```python
from build123d import *

# Parameters (mm, degrees)
CROQUIS1_R              = 3
SALIENTE_EXTRUIR1_DEPTH = 5
CHAFL_N1_SIZE           = 2


with BuildPart() as part:
    # Croquis1 → Saliente-Extruir1 (new body)
    with BuildSketch(Plane(origin=(0, 0, 0), x_dir=(1, 0, 0), z_dir=(0, 1, 0))):
        Polygon((-149.607843137, -39.607843137), (-129.607843137, -19.607843137), (170.392156863, -19.607843137), (190.392156863, -39.607843137), (220.392156863, -39.607843137), (220.392156863, 40.392156863), (-179.607843137, 40.392156863), (-179.607843137, -39.607843137), align=None)
        with Locations(Location((-164.607843137, 20.392156863, 0), (0, 0, 270))):
            Circle(CROQUIS1_R, mode=Mode.SUBTRACT)
        with Locations(Location((-99.607843137, 30.392156863, 0), (0, 0, 270))):
            Circle(CROQUIS1_R, mode=Mode.SUBTRACT)
        with Locations(Location((140.392156863, 30.392156863, 0), (0, 0, 270))):
            Circle(CROQUIS1_R, mode=Mode.SUBTRACT)
        with Locations(Location((20.392156863, 30.392156863, 0), (0, 0, 270))):
            Circle(CROQUIS1_R, mode=Mode.SUBTRACT)
        with Locations(Location((-164.607843137, -19.607843137, 0), (0, 0, 270))):
            Circle(CROQUIS1_R, mode=Mode.SUBTRACT)
        with Locations(Location((205.392156863, 20.392156863, 0), (0, 0, 270))):
            Circle(CROQUIS1_R, mode=Mode.SUBTRACT)
        with Locations(Location((205.392156863, -19.607843137, 0), (0, 0, 270))):
            Circle(CROQUIS1_R, mode=Mode.SUBTRACT)
    extrude(amount=SALIENTE_EXTRUIR1_DEPTH)

    # Chaflán1
    chafl_n1_edges = [part.edges().sort_by_distance(p)[0] for p in [
        (-139.607843137, 5, 29.607843137),
        (20.392156863, 5, 19.607843137),
        (180.392156863, 5, 29.607843137),
        (205.392156863, 5, 39.607843137),
        (220.392156863, 5, -0.392156863),
        (20.392156863, 5, -40.392156863),
        (-179.607843137, 5, -0.392156863),
        (-164.607843137, 5, 39.607843137),
    ]]
    chamfer(chafl_n1_edges, length=CHAFL_N1_SIZE)


solid = part.part
```
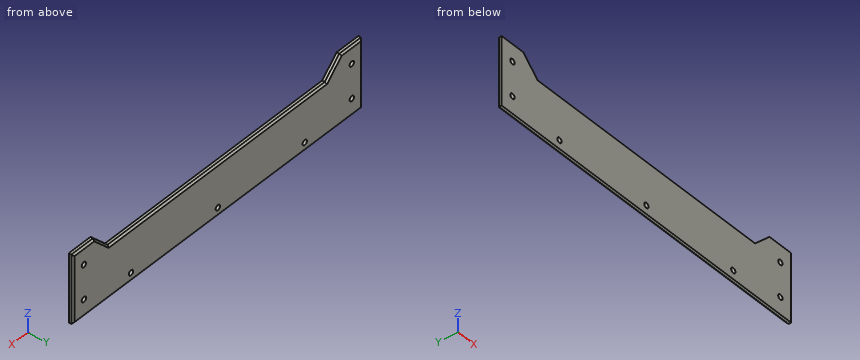
Geometry check sheet. Reference: the model listing, model coordinates, mm. Coordinates: 2 decimals unless noted, no trailing zeros. Order: outer loops, then holes, each group sorted by start corner. A loop starts at its lowest first (then second) coordinate and runs counter-clockwise, first axis right, second up.
Item 1: Scan lines: line 1 along X through (y, z) = (0.65, -30.5); line 2 along Z through (x, y) = (160, 1.25); line 3 along X through (y, z) = (4.5, -28.5). Record each from-to range of solid material in increasing order.
Item 2: Section check B-B (x = -80). Enter the section's corners in (y, z), plus the area to 3 significant figures.
Item 3: Section check A-A (y = 1.1). Enter the section's corners in (x, z), plus the area to 3 significant figures.
Item 4: Depth check by flat-ended pin: pin 1 (7 mm diameter, centred on x = -99.61, z = -30.39, fed in from -Y); pin 2 (1.5 mm diameter, centred on x = 34.5, y = 2, fed in from +Z). Enter the tip coordinate at first touch or a pass-through.
Item 5: Section check C-C (z = 26.5). Enter the section's corners in (x, y), plus the area to 3 significant figures.
Check sheet entries:
1. line 1: x = -179.61 to -102.61, -96.61 to 17.39, 23.39 to 137.39, 143.39 to 220.39
1. line 2: z = -40.39 to 19.61
1. line 3: x = -178.11 to -101.94, -97.28 to 18.06, 22.72 to 138.06, 142.72 to 218.89
2. outline: (0, -40.39) - (3, -40.39) - (5, -38.39) - (5, 17.61) - (3, 19.61) - (0, 19.61) - close
2. area: 296 mm2
3. outline: (-179.61, -40.39) - (220.39, -40.39) - (220.39, 39.61) - (190.39, 39.61) - (170.39, 19.61) - (-129.61, 19.61) - (-149.61, 39.61) - (-179.61, 39.61) - close; hole circle Ø6 at (-164.61, -20.39); hole circle Ø6 at (-164.61, 19.61); hole circle Ø6 at (-99.61, -30.39); hole circle Ø6 at (20.39, -30.39); hole circle Ø6 at (140.39, -30.39); hole circle Ø6 at (205.39, -20.39); hole circle Ø6 at (205.39, 19.61)
3. area: 25,400 mm2
4. pin 1: stops at y = 0
4. pin 2: stops at z = 19.61
5. outline: (-179.61, 0) - (-136.5, 0) - (-136.5, 3) - (-139.33, 5) - (-177.61, 5) - (-179.61, 3) - close; (177.28, 0) - (220.39, 0) - (220.39, 3) - (218.39, 5) - (180.11, 5) - (177.28, 3) - close
5. area: 421 mm2
